```python
from build123d import *

# Parameters (mm, degrees)
F0_R     = 3.96875
F0_R_2   = 2.15265
F1_DEPTH = 3.175


with BuildPart() as f1:
    # F0 (on Top) → F1 (new body)
    with BuildSketch(Plane.XY):
        with BuildLine():
            Line((31.75, 28.964184), (22.225, 28.964184))
            Line((22.225, 28.964184), (-5.752253, 21.467701))
            ThreePointArc((-5.752253, 21.467701), (-22.225, 0), (-5.752253, -21.467701))
            Line((-5.752253, -21.467701), (22.225, -28.964184))
            Line((22.225, -28.964184), (31.75, -28.964184))
            Line((31.75, -28.964184), (31.75, 28.964184))
        make_face()
        with Locations((-11.786586, -11.786586)):
            Circle(F0_R, mode=Mode.SUBTRACT)
        with Locations((0, -9.525)):
            Circle(F0_R_2, mode=Mode.SUBTRACT)
        with Locations((11.786586, -11.786586)):
            Circle(F0_R_2, mode=Mode.SUBTRACT)
        with Locations((-11.786586, 11.786586)):
            Circle(F0_R_2, mode=Mode.SUBTRACT)
        Circle(F0_R, mode=Mode.SUBTRACT)
        with Locations((0, 9.525)):
            Circle(F0_R_2, mode=Mode.SUBTRACT)
        with Locations((11.786586, 11.786586)):
            Circle(F0_R, mode=Mode.SUBTRACT)
    extrude(amount=F1_DEPTH)


solid = f1.part
```
Could you check a few things on this model? Use its own coordinates, in mm. Round coordinates to 2 decimals unless told otherwise and drop trailing zeros. Write each loop counter-clockwise with the first axis right and the second up, starting at its lowest first coordinate (ties: lowest second). Pieces come first, ordered by that corner, then holes. Notation, with made-up numbers: M -13,56.25 L 5,56.25 A13 cw 5,67.25 Z; hole C -39.5,39 d11. An arc over 180 degrees is marked long. Answer in a Markdown table with one row per item. Add a question column.
Q1. If I drill on line 1 (Y direction, x = -12.5, z = 1.1); line 2 (X direction, y = 13, z = 1.6); line 3 (X direction, y = -10.5, z = 1.75), over which ranges is the centre line in solid material (lowest first)? Write a range as from..to.
Q2. Imagine slicing it at A-A (y = 0). Please give me the cut outline in (x, z) (3 decimals), then the cut area to 3 significant figures.
Q3. Will these pins go through, and if not, where does the flat tip stop? pin 1 Ø3.5 at (x, y) = (-11.79, 11.79) entering from -Z; pin 2 Ø5.5 at (x, y) = (0, 9.525) entering from +Z (3 decimals); pin 3 Ø1 at (x, z) = (6.5, 1) entering from +Y.
Q4. Imagine slicing it at C-C (y = -11). Please give me the cut outline in (x, z) (3 decimals).
Q5. If we mould it in two halves opening along X, with no side actions, what happens to faces 1 (the flat face through (31.75, 0, 2)), 2 (the cylindrical face through (-0.28, 11.66, 1.57)), 3 (the flat face through (27, 28.964, 2)), 4 (the cylindrical face through (-0.86, -3.874, 1.565))? For each: +X half, -X half, draft (parallel to the pull), parting line (faces both ways), or undercut.
Q6. Imagine slicing it at D-D (z = 2.3). Give the number of separate pieces and of enclosed holes in the cut face, then the cut area to 3 significant figures.
Q7. Imagine slicing it at B-B (x = 0). Please give me the cut outline in (y, z) (3 decimals), then the cut area to 3 significant figures.
Values:
| question | item | result |
|---|---|---|
| 1 | line 1 | -18.38..-15.69, -7.88..9.76, 13.82..18.38 |
| 1 | line 2 | -18.03..-13.56, -10.01..8.01, 15.57..31.75 |
| 1 | line 3 | -19.59..-15.54, -8.03..-1.92, 1.92..10.06, 13.51..31.75 |
| 2 | outline | M -22.225,0 L -3.969,0 L -3.969,3.175 L -22.225,3.175 Z; M 3.969,0 L 31.75,0 L 31.75,3.175 L 3.969,3.175 Z |
| 2 | area | 146 mm^2 |
| 3 | pin 1 | through |
| 3 | pin 2 | z = 3.175 |
| 3 | pin 3 | y = 24.88 |
| 4 | outline | M -19.312,0 L -15.677,0 L -15.677,3.175 L -19.312,3.175 Z; M -7.897,0 L -1.568,0 L -1.568,3.175 L -7.897,3.175 Z; M 1.568,0 L 9.783,0 L 9.783,3.175 L 1.568,3.175 Z; M 13.79,0 L 31.75,0 L 31.75,3.175 L 13.79,3.175 Z |
| 5 | face 1 | +X half |
| 5 | face 2 | undercut |
| 5 | face 3 | draft |
| 5 | face 4 | undercut |
| 6 | separate pieces | 1 |
| 6 | enclosed holes | 7 |
| 6 | area | 2,280 mm^2 |
| 7 | outline | M -23.009,0 L -11.678,0 L -11.678,3.175 L -23.009,3.175 Z; M -7.372,0 L -3.969,0 L -3.969,3.175 L -7.372,3.175 Z; M 3.969,0 L 7.372,0 L 7.372,3.175 L 3.969,3.175 Z; M 11.678,0 L 23.009,0 L 23.009,3.175 L 11.678,3.175 Z |
| 7 | area | 93.6 mm^2 |
